```python
from build123d import *

# Parameters (mm, degrees)
F0_R     = 12.7
F0_R_2   = 6.35
F1_DEPTH = 25.4
F2_R     = 3.3782
F3_DEPTH = 6.35
F4_R     = 12.7
F4_R_2   = 11.1125
F5_DEPTH = 25.4
F6_R     = 4.2799
F7_DEPTH = 25.4


with BuildPart() as f1:
    # F0 (on Front) → F1 (new body)
    with BuildSketch(Plane.XZ):
        Circle(F0_R)
        Circle(F0_R_2, mode=Mode.SUBTRACT)
    extrude(amount=F1_DEPTH)

    # F4 (on face) → F5 (cut)
    with BuildSketch(Plane.XZ.offset(6.35)):
        Circle(F4_R)
        Circle(F4_R_2, mode=Mode.SUBTRACT)
    extrude(amount=F5_DEPTH, mode=Mode.SUBTRACT)


with BuildPart() as f3:
    # F2 (on Front) → F3 (new body)
    with BuildSketch(Plane.XZ):
        Circle(F2_R)
    extrude(amount=F3_DEPTH)

    # F6 (on face) → F7 (cut)
    with BuildSketch(Plane.XZ.offset(6.35)):
        Circle(F6_R)
    extrude(amount=-F7_DEPTH, mode=Mode.SUBTRACT)


solid = f1.part
```
Input: part model. Units: mm. Frame: model coordinates. A direction names the side the tool comes from. Give positions to 0.01 mm unless a question says otherwise; leave off trailing zeros. Order: outer loops, then holes, each group sorted by start corner. A loop starts at its lowest first (then second) coordinate and runs counter-clockwise, first axis right, second up.
1. Pin query (flat end, axial travel): pin 1 (11.5 mm diameter, centred on x = 0, z = 0, fed in from +Y); pin 2 (4 mm diameter, centred on y = -22, z = -3, fed in from -X); pin 3 (6 mm diameter, centred on y = -14, z = 6, fed in from -X); pin 4 (1 mm diameter, centred on y = -12.5, z = -5, fed in from -X). Return the tip coordinate at first contact, or that it passes through.
Derived:
pin 1: passes through
pin 2: stops at x = -11.07
pin 3: stops at x = -10.7
pin 4: stops at x = -10.16
2. Section A-A on x = 0. Return the cut outline in (y, z), and give its area (3 significant figures).
Derived:
outline: (-25.4, -11.11) - (-6.35, -11.11) - (-6.35, -12.7) - (0, -12.7) - (0, -6.35) - (-25.4, -6.35) - close; (-25.4, 6.35) - (0, 6.35) - (0, 12.7) - (-6.35, 12.7) - (-6.35, 11.11) - (-25.4, 11.11) - close
area: 262 mm2
3. Mould query, pull axis X, two halves, no side actions, for faces 1 (the flat face through (5, -25.4, -5)), 2 (the cylindrical face through (-1.38, -12.52, -6.2)), 3 (the cylindrical face through (10.6, -15.74, 3.34)). Classes: released by +X, released by -X, zero draft, split by the parting line, or undercut.
Derived:
face 1: zero draft
face 2: undercut
face 3: split by the parting line
4. Reachability of faces 4 (the flat face through (0.88, -6.35, -11.23)), 5 (the cylindrical face through (-2.75, -3.13, -12.4)) from +Z, -Z, +X, -X, +Y, -Y: full face, straight path, thin tool, end or side. Return the list, or none.
Derived:
face 4: -Y
face 5: +Y, -Y
5. Section C-C on y = -3.5. Return the cut outline in (x, z), and give its area (3 significant figures).
Derived:
outline: circle Ø25.4 at (0, 0); hole circle Ø12.7 at (0, 0)
area: 380 mm2
6. Section D-D on x = 7.5. Return the cut outline in (y, z), and give its area (3 significant figures).
Derived:
outline: (-25.4, -8.2) - (-6.35, -8.2) - (-6.35, -10.25) - (0, -10.25) - (0, 10.25) - (-6.35, 10.25) - (-6.35, 8.2) - (-25.4, 8.2) - close
area: 443 mm2
7. Material intervals for L1, parallel to Z at x = 0, y = -12; L2, parallel to Z at x = 0, y = -4; L3, parallel to X at y = -16.75, z = 1.75, sorted ascending.
Derived:
L1: z = -11.11 to -6.35, 6.35 to 11.11
L2: z = -12.7 to -6.35, 6.35 to 12.7
L3: x = -10.97 to -6.1, 6.1 to 10.97
8. Section B-B on z = 0. Return the cut outline in (x, y).
Derived:
outline: (-12.7, -6.35) - (-11.11, -6.35) - (-11.11, -25.4) - (-6.35, -25.4) - (-6.35, 0) - (-12.7, 0) - close; (6.35, -25.4) - (11.11, -25.4) - (11.11, -6.35) - (12.7, -6.35) - (12.7, 0) - (6.35, 0) - close
